```python
from build123d import *

# Parameters (mm, degrees)
SZKIC1_W                    = 26
SZKIC1_H                    = 44
DODANIE_WYCI_GNI_CIE1_DEPTH = 7
SZKIC2_R                    = 2.15
WYTNIJ_WYCI_GNI_CIE1_DEPTH  = 5
ZAOKR_GLENIE1_R             = 2


with BuildPart() as part:
    # Szkic1 → Dodanie-wyciągnięcie1 (new body)
    with BuildSketch(Plane(origin=(0, 0, 0), x_dir=(1, 0, 0), z_dir=(0, 1, 0))):
        Rectangle(SZKIC1_W, SZKIC1_H)
    extrude(amount=DODANIE_WYCI_GNI_CIE1_DEPTH)

    # Szkic2 → Wytnij-wyciągnięcie1 (cut)
    with BuildSketch(Plane.XY.offset(22)):
        with Locations((-8.68, 3.5)):
            Circle(SZKIC2_R)
        with Locations(Location((8.68, 3.5, 0), (0, 0, 180))):
            Circle(SZKIC2_R)
    wytnij_wyci_gni_cie1 = extrude(amount=-WYTNIJ_WYCI_GNI_CIE1_DEPTH, mode=Mode.SUBTRACT)

    # Lustro1: Wytnij-wyciągnięcie1 across plane
    add(wytnij_wyci_gni_cie1.mirror(Plane.XY), mode=Mode.SUBTRACT)

    # Zaokrąglenie1
    zaokr_glenie1_edges = [part.edges().sort_by_distance(p)[0] for p in [
        (-13, 7, 0),
        (13, 7, 0),
        (-13, 0, 0),
        (13, 0, 0),
    ]]
    fillet(zaokr_glenie1_edges, radius=ZAOKR_GLENIE1_R)


solid = part.part
```
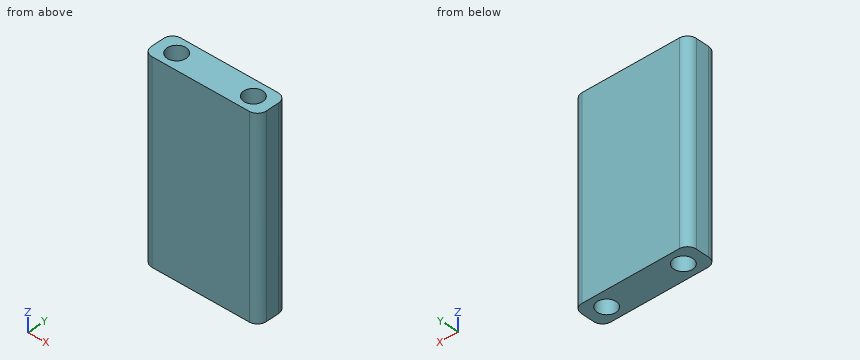
Model file for the job. Use its own axes, mm. Give positions to 0.01 mm unless a question says otherwise; leave off trailing zeros. Loops run counter-clockwise (first coordinate to the right, second up) from the corner with the lowest first, then second, coordinate; pieces in that order, holes last. Notation, with made-up numbers: (14, 61) -> (60, 61) arc R23 ccw to (60, 85) -> close; hole circle Ø7 at (76.5, -11.75). An arc over 180 degrees is marked (long way). Write each question's results on one line, items separated by ' | '.
(1) Cut at C-C on z = 1. List the corners of the cut face in (x, y).
Geometry results:
outline: (-13, 2) arc R2 ccw to (-11, 0) -> (11, 0) arc R2 ccw to (13, 2) -> (13, 5) arc R2 ccw to (11, 7) -> (-11, 7) arc R2 ccw to (-13, 5) -> close
(2) Flat gauge pins, fed straight in: pin 1 Ø3.5 at (x, y) = (9.5, 2.5) entering from +Z; pin 2 Ø1.3 at (x, y) = (9.5, 4.5) entering from -Z; pin 3 Ø3.5 at (x, y) = (8.68, 3.5) entering from +Z. Where does each tip first touch, or does it go through?
Geometry results:
pin 1: stops at z = 22 | pin 2: stops at z = -17 | pin 3: stops at z = 17
(3) Probe line 1 along Y through (x, z) = (8.68, 20.05); line 2 along X through (y, z) = (4.25, -19); line 3 along Z through (x, y) = (-9.75, 3.25). List the from-to ranges inside material, lowest first.
Geometry results:
line 1: y = 0 to 1.35, 5.65 to 7 | line 2: x = -13 to -10.69, -6.67 to 6.67, 10.69 to 13 | line 3: z = -17 to 17
(4) Cut at A-A on x = 8.68. List the corners of the cut face in (y, z), and give its area (3 significant figures).
Geometry results:
outline: (0, -22) -> (1.35, -22) -> (1.35, -17) -> (5.65, -17) -> (5.65, -22) -> (7, -22) -> (7, 22) -> (5.65, 22) -> (5.65, 17) -> (1.35, 17) -> (1.35, 22) -> (0, 22) -> close | area: 265 mm²
(5) Cut at B-B on y = 3.5. List the corners of the cut face in (x, z).
Geometry results:
outline: (-13, -22) -> (-10.83, -22) -> (-10.83, -17) -> (-6.53, -17) -> (-6.53, -22) -> (6.53, -22) -> (6.53, -17) -> (10.83, -17) -> (10.83, -22) -> (13, -22) -> (13, 22) -> (10.83, 22) -> (10.83, 17) -> (6.53, 17) -> (6.53, 22) -> (-6.53, 22) -> (-6.53, 17) -> (-10.83, 17) -> (-10.83, 22) -> (-13, 22) -> close
(6) Cut at D-D on x = -7.5. List the corners of the cut face in (y, z), and give its area (3 significant figures).
Geometry results:
outline: (0, -22) -> (1.7, -22) -> (1.7, -17) -> (5.3, -17) -> (5.3, -22) -> (7, -22) -> (7, 22) -> (5.3, 22) -> (5.3, 17) -> (1.7, 17) -> (1.7, 22) -> (0, 22) -> close | area: 272 mm²
